Autodesk Inventor part; units mm, degrees
ref_plane "YZ Plane" through (0, 0, 0) normal (1, 0, 0) x (0, 1, 0)
ref_plane "XZ Plane" through (0, 0, 0) normal (0, 1, 0) x (-1, 0, 0)
ref_plane "XY Plane" through (0, 0, 0) normal (0, 0, 1) x (1, 0, 0)
sketch "Sketch1" plane through (0, 0, 0) normal (1, 0, 0) x (0, 1, 0)
  line L0 (0, 0) -> (0, 36)
  line L1 (0, 36) -> (6, 36)
  line L2 (6, 36) -> (6, 6)
  line L3 (6, 6) -> (36, 6)
  line L4 (36, 6) -> (36, 0)
  line L5 (36, 0) -> (0, 0)
  dimension "d0" = 36
  dimension "d1" = 6
  dimension "d2" = 30
  dimension "d3" = 30
  dimension "d4" = 6
  dimension "d5" = 36
extrude "Extrusion1" add sketch "Sketch1" against normal blind 36
sketch "Sketch2" plane through (0, 6, 36) normal (0, 1, 0) x (1, 0, 0)
  circle A0 centre (-28, 15) radius 3.25
  circle A1 centre (-8, 15) radius 3.25
  line L0 (0, 0) -> (-36, 0)
  line L1 (0, 30) -> (0, 0)
  line L2 (-36, 0) -> (-36, 30)
  line L3 (-36, 30) -> (3.723, 30) construction
  point P0 (0, 36)
  point P1 (-5.4498, 30)
  dimension "d8" = 6.5
  dimension "d9" = 6.5
  dimension "d10" = 20
  dimension "d11" = 15
  dimension "d12" = 15
  dimension "d13" = 8
sketch "Sketch3" plane through (0, 6, 6) normal (0, 0, 1) x (1, 0, 0)
  circle A0 centre (-28, 15) radius 3.25
  line L0 (-36, 0) -> (-36, 30)
  line L1 (0, 30) -> (-36, 30)
  circle A1 centre (-8, 15) radius 3.25
  point P0 (0, -6)
  dimension "d14" = 6.5
  dimension "d15" = 8
  dimension "d16" = 15
  dimension "d17" = 6.5
  dimension "d18" = 20
extrude "Extrusion2" cut sketch "Sketch3" against normal blind 6
extrude "Extrusion3" cut sketch "Sketch2" against normal blind 6
properties part number "Normal_Connector"
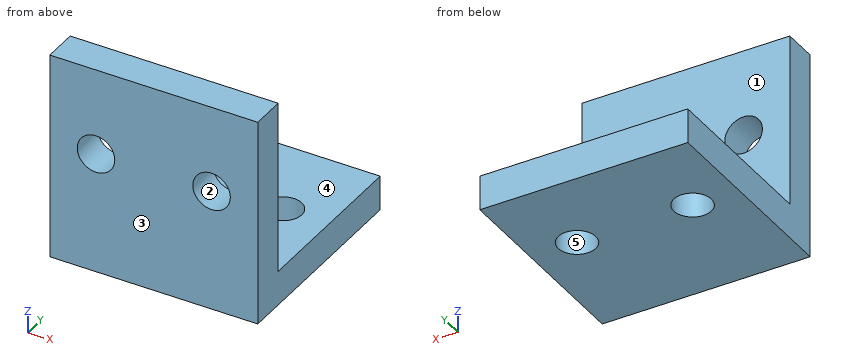
Can you work these out from the model? Positions are in its coordinate system, mm. Face numbers are marked on the shaded views. A direction names the side the tool comes from. Give positions to 0.01 mm unless a question says otherwise; leave off trailing zeros. Order: outer loops, then holes, each group sorted by start corner. A loop starts at its lowest first (then second) coordinate and runs counter-clockwise, first axis right, second up. Notation, with made-up numbers: M -28,27 L -1,27 A19 cw -1,44 Z; hole C -24.5,-6 d10. An arc over 180 degrees is marked long. Write item = value, one per line. Start each with the question number.
Q1. We'd pull the mould along Y, two halves only. Please class the marked faces 3, 4 and 5: pulls with the +Y half, pulls with the -Y half, needs draft (parallel to the pull), parting line crosses it, or undercut.
Q2. Will this pin go through, and if not, where does the flat tip stop? pin 1 Ø6 at (x, z) = (-31.5, 28) entering from +Y.
Q3. Suppose I cut it at A-A (x = -28). Write out the boundary of the cut face in (y, z).
Q4. For the marked faces 1 and 2, which set-ups out of +Z, -Z, +X, -X, +Y, -Y let a thin tool reach every point of the face, with its end or its side?
Q5. Suppose I cut it at C-C (y = 21). Write out the boundary of the cut face in (x, z).
Q6. I need wall thicknesses on probe 1 along X at (y, z) = (2.25, 21); probe 2 along Y at (x, z) = (-8, 2.9); probe 3 along Z at (x, y) = (-25, 8). Which ranges of each line are inside material? Lowest first, please. Write a range as [from, to].
Q7. Suppose I cut it at B-B (z = 5). Write out the boundary of the cut face in (x, y).
Check result:
q1.face_3 = pulls with the -Y half
q1.face_4 = needs draft
q1.face_5 = undercut
q2.pin_1 = 6
q3.outline = M 0,0 L 17.75,0 L 17.75,6 L 6,6 L 6,17.75 L 0,17.75 Z; M 0,24.25 L 6,24.25 L 6,36 L 0,36 Z; M 24.25,0 L 36,0 L 36,6 L 24.25,6 Z
q4.face_1 = +Z, +X, -X, +Y
q4.face_2 = +Y, -Y
q5.outline = M -36,0 L -31.25,0 L -31.25,6 L -36,6 Z; M -24.75,0 L -11.25,0 L -11.25,6 L -24.75,6 Z; M -4.75,0 L 0,0 L 0,6 L -4.75,6 Z
q6.probe_1 = [-36, -31.25], [-24.75, -11.25], [-4.75, 0]
q6.probe_2 = [0, 17.75], [24.25, 36]
q6.probe_3 = [0, 6]
q7.outline = M -36,0 L 0,0 L 0,36 L -36,36 Z; hole C -28,21 d6.5; hole C -8,21 d6.5
